Here's how the part is built. I have some questions about the finished solid (model axes, mm). Face numbers are marked on the shaded views. Round coordinates to 2 decimals unless told otherwise and drop trailing zeros. Loops run counter-clockwise (first coordinate to the right, second up) from the corner with the lowest first, then second, coordinate; pieces in that order, holes last. Notation, with made-up numbers: (-6, 59) -> (48, 59) arc R25 ccw to (48, 92) -> close; hole circle Ø11 at (89.5, 57.25). An arc over 180 degrees is marked (long way). One line per item, written item: value. Start each with the question number.
```python
from build123d import *

# Parameters (mm, degrees)
BOSS_EXTRUDE1_DEPTH = 18
SKETCH3_R           = 3
CUT_EXTRUDE1_DEPTH  = 35.5
CHAMFER2_SIZE       = 2


with BuildPart() as part:
    # Sketch1 → Boss-Extrude1 (new body)
    with BuildSketch(Plane.XY):
        Polygon((0, 0), (3.5, 0), (3.5, 2.5), (6, 2.5), (6, 5), (8.5, 5), (8.5, 7.5), (11, 7.5), (11, 10), (13.5, 10), (13.5, 12.5), (16, 12.5), (16, 15), (18.5, 15), (18.5, 12.5), (21, 12.5), (21, 10), (23.5, 10), (23.5, 7.5), (26, 7.5), (26, 5), (28.5, 5), (28.5, 2.5), (31, 2.5), (31, 0), (34.5, 0), (34.5, 60), (0, 60), align=None)
    extrude(amount=BOSS_EXTRUDE1_DEPTH)

    # Sketch2 → Cut-Revolve1 (revolve, cut)
    with BuildSketch(Plane.XY.offset(9)):
        Polygon((11.25, 60), (11.25, 40), (17.25, 36.535898385), (17.25, 60), align=None)
    revolve(axis=Axis((17.25, 60, 9), (0, -1, 0)), mode=Mode.SUBTRACT)

    # Sketch3 → Cut-Extrude1 (cut, through all)
    with BuildSketch(Plane(origin=(34.5, 0, 0), x_dir=(0, 0, -1), z_dir=(1, 0, 0))):
        with Locations((-9, 53)):
            Circle(SKETCH3_R)
    extrude(amount=-CUT_EXTRUDE1_DEPTH, mode=Mode.SUBTRACT)

    # Chamfer2
    chamfer2_edges = [part.edges().sort_by_distance(p)[0] for p in [
        (17.25, 60, 18),
        (17.25, 60, 0),
        (0, 60, 9),
        (34.5, 60, 9),
    ]]
    chamfer(chamfer2_edges, length=CHAMFER2_SIZE)


solid = part.part
```
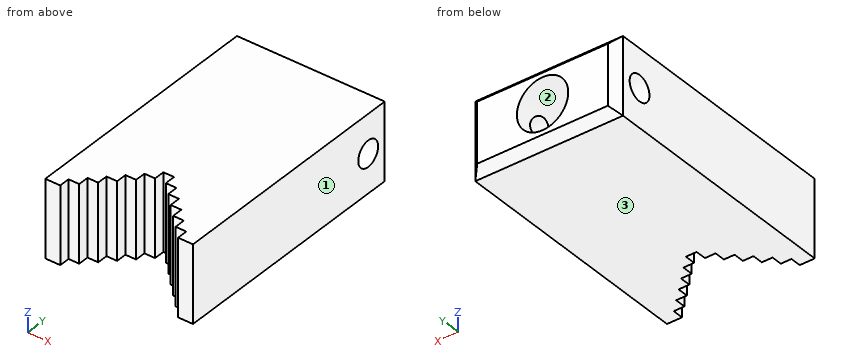
Q1. I want a section at B-B on x = 24.5. Please give me the cut outline in (y, z).
Q2. If we mould it in two halves opening along X, with no side actions, what happens to the marked faces 1, 2 and 3? For each: released by +X, released by -X, zero draft, split by the parting line, or undercut.
Q3. If I drill on line 1 along Z through (x, y) = (4.5, 53); line 2 along X through (y, z) = (10.5, 14.25); line 3 along X through (y, z) = (7, 9), over which ranges is the centre line in solid material (lowest first)?
Q4. Will these pins go through, and if not, where does the flat tip stop? P1, Ø0.8, axis at x = 20, z = 7.5, coming from the -Y side; P2, Ø2, axis at x = 24.5, z = 5.5, coming from the -Y side; P3, Ø0.8, axis at x = 27.5, z = 13, coming from the -Y side.
Q5. I want a section at A-A on y = 53. Please give me the cut outline in (x, z).
Q6. I want a section at C-C on y = 42.5. Please give me the cut outline in (x, z).
Answers below:
1. outline: (7.5, 0) -> (58, 0) -> (60, 2) -> (60, 16) -> (58, 18) -> (7.5, 18) -> close; hole circle Ø6 at (53, 9)
2. face 1: released by +X
2. face 2: undercut
2. face 3: zero draft
3. line 1: z = 0 to 6, 12 to 18
3. line 2: x = 0 to 13.5, 21 to 34.5
3. line 3: x = 0 to 8.5, 26 to 34.5
4. P1: stops at y = 12.5
4. P2: stops at y = 7.5
4. P3: stops at y = 5
5. outline: (0, 0) -> (34.5, 0) -> (34.5, 6) -> (22.45, 6) arc R6 cw to (12.05, 6) -> (0, 6) -> close; (0, 12) -> (12.05, 12) arc R6 cw to (22.45, 12) -> (34.5, 12) -> (34.5, 18) -> (0, 18) -> close
6. outline: (0, 0) -> (34.5, 0) -> (34.5, 18) -> (0, 18) -> close; hole circle Ø12 at (17.25, 9)
